Build history of the part. All positions in model axes, mm. A direction names the side the tool comes from. Coordinates: 2 decimals unless noted, no trailing zeros. Loops run counter-clockwise (first coordinate to the right, second up) from the corner with the lowest first, then second, coordinate; pieces in that order, holes last.
(1) Slice it at C-C (z = 220). Give the cut face in (x, y), and give its area (3 significant figures).
(2) Tool access for faces 1 (the face through (-4.8, -8.2, 143.3)), 2 (the face through (-6, 5, 265)), 3 (the face through (-7.493, 0.33, 12.675)): list every direction of +Z, -Z, +X, -X, +Y, -Y with a clear straight run to the whole face (end or side of a thin tool).
(3) Slice it at A-A (y = 0). Give the cut face in (x, z).
(4) Flat gauge pins, fed straight in: P1, Ø1, axis at x = 1, z = 174.5, coming from the +Y side; P2, Ø6, axis at x = -4.5, z = 230, coming from the -Y side; P3, Ø6, axis at x = -1.5, z = 124.5, coming from the +Y side. Where does each tip first touch, or does it go through?
(5) Slice it at B-B (x = 4.5). Give the cut face in (y, z), and give its area (3 significant figures).
(6) Wall check: L1, parallel to Z at x = 2, y = -8; L2, parallel to Y at x = -2.5, z = 146; L3, parallel to X at y = -7.5, z = 86. Give the ranges that are in metal, low to high.
(7) Two-plate mould, pull along X, no slides. Class faces 4 (the face through (-6, 5, 25)), 5 (the face through (4.8, 8.2, 143.3)), 6 (the face through (-4.684, 8.266, 143.32)): pulls with the +X half, pulls with the -X half, needs draft (parallel to the pull), parting line crosses it, or undercut.
from build123d import *

# Parameters (mm, degrees)
BOSS_EXTRU_1_DEPTH      = 320
ESQUISSE2_R             = 10.969655115
ESQUISSE2_R_2           = 7.5
ENL_V_MAT_EXTRU_1_DEPTH = 55
ENL_V_START             = -295
ESQUISSE2_2_R           = 10.969655115
ESQUISSE2_2_R_2         = 7.5
ENL_V_MAT_EXTRU_2_DEPTH = 25


with BuildPart() as part:
    # Esquisse1 → Boss.-Extru.1 (new body)
    with BuildSketch(Plane.XY):
        Polygon((9.5, -5.484827557), (9.5, 5.484827557), (0, 10.969655115), (-9.5, 5.484827557), (-9.5, -5.484827557), (0, -10.969655115), align=None)
    extrude(amount=BOSS_EXTRU_1_DEPTH)

    # Esquisse2 → Enlèv. mat.-Extru.1 (cut)
    with BuildSketch(Plane.XY.offset(320)):
        Circle(ESQUISSE2_R)
        Circle(ESQUISSE2_R_2, mode=Mode.SUBTRACT)
    extrude(amount=-ENL_V_MAT_EXTRU_1_DEPTH, mode=Mode.SUBTRACT)

    # Esquisse2<2> → Enlèv. mat.-Extru.2 (cut)
    with BuildSketch(Plane.XY.offset(320).offset(ENL_V_START)):
        Circle(ESQUISSE2_2_R)
        Circle(ESQUISSE2_2_R_2, mode=Mode.SUBTRACT)
    extrude(amount=-ENL_V_MAT_EXTRU_2_DEPTH, mode=Mode.SUBTRACT)


solid = part.part
Response values:
1. outline: (-9.5, -5.48) - (0, -10.97) - (9.5, -5.48) - (9.5, 5.48) - (0, 10.97) - (-9.5, 5.48) - close
1. area: 313 mm2
2. face 1: +Z, -Z, -X, -Y
2. face 2: +Z
2. face 3: -Z
3. outline: (-9.5, 25) - (-7.5, 25) - (-7.5, 0) - (7.5, 0) - (7.5, 25) - (9.5, 25) - (9.5, 265) - (7.5, 265) - (7.5, 320) - (-7.5, 320) - (-7.5, 265) - (-9.5, 265) - close
4. P1: stops at y = 10.68
4. P2: stops at y = -10.1
4. P3: stops at y = 10.97
5. outline: (-8.37, 25) - (-6, 25) - (-6, 0) - (6, 0) - (6, 25) - (8.37, 25) - (8.37, 265) - (6, 265) - (6, 320) - (-6, 320) - (-6, 265) - (-8.37, 265) - close
5. area: 4,980 mm2
6. L1: z = 25 to 265
6. L2: y = -9.53 to 9.53
6. L3: x = -6.01 to 6.01
7. face 4: needs draft
7. face 5: pulls with the +X half
7. face 6: pulls with the -X half
